Autodesk Inventor part; units mm, degrees
ref_plane "YZ Plane" through (0, 0, 0) normal (1, 0, 0) x (0, 1, 0)
ref_plane "XZ Plane" through (0, 0, 0) normal (0, 1, 0) x (-1, 0, 0)
ref_plane "XY Plane" through (0, 0, 0) normal (0, 0, 1) x (1, 0, 0)
sketch "Sketch1" plane through (0, 0, 0) normal (1, 0, 0) x (0, 1, 0)
  line L0 (-19.05, 19.05) -> (19.05, 19.05)
  line L1 (19.05, 19.05) -> (19.05, -19.05)
  line L2 (19.05, -19.05) -> (-19.05, -19.05)
  line L3 (-19.05, -19.05) -> (-19.05, 19.05)
  line L4 (-19.05, 19.05) -> (19.05, -19.05) construction
  line L5 (19.05, 19.05) -> (-19.05, -19.05) construction
  line L6 (19.05, 19.05) -> (-19.05, -19.05)
  line L7 (19.05, -19.05) -> (-19.05, 19.05)
  line L8 (0, 0) -> (0, -19.05)
  line L9 (0, 0) -> (0, 19.05)
  circle A0 centre (0, 9.525) radius 3.81
  circle A1 centre (0, -9.525) radius 3.81
  dimension "d0" = 38.1
  dimension "d1" = 38.1
  dimension "d2" = 7.62
  dimension "d3" = 7.62
  dimension "d4" = 19.05
extrude "Extrusion1" add sketch "Sketch1" along normal blind 38.1 contours L7 L6 L3 | L0 L9 A0 L7 | L0 L6 L9 A0 | L6 L8 A1 L2 | L6 L1 L7 | L7 L2 L8 A1
sketch "Sketch2" plane through (0, -19.05, -19.05) normal (0, -1, 0) x (1, 0, 0)
  line L0 (38.1, 0) -> (38.1, 38.1)
  line L1 (0, 0) -> (38.1, 0)
  line L2 (38.1, 38.1) -> (38.1, 0)
  line L3 (38.1, 0) -> (0, 0)
  line L4 (0, 0) -> (0, 38.1)
  line L5 (0, 0) -> (0, 38.1)
  line L6 (0, 38.1) -> (38.1, 38.1)
  line L7 (0, 38.1) -> (38.1, 38.1)
  line L8 (0, 0) -> (38.1, 38.1)
  line L9 (38.1, 0) -> (0, 38.1)
  circle A0 centre (19.05, 19.05) radius 12.5
  point P0 (0, 19.05)
  dimension "d7" = 25
extrude "Extrusion2" cut sketch "Sketch2" against normal blind 15 contours A0 L8 L9 | L9 L8 A0 | L8 L9 A0 | A0 L9 L8
fillet "Fillet1" radius 2 1 edges at (19.05, 19.05, 19.05)
fillet "Fillet2" radius 2 1 edges at (19.05, 19.05, -19.05)
properties part number "cube fixation2"
Check sheet for the modelled part. Datum: model origin and axes. Units: mm. A direction names the side the tool comes from. Round coordinates to 2 decimals unless told otherwise and drop trailing zeros. Order: outer loops, then holes, each group sorted by start corner. A loop starts at its lowest first (then second) coordinate and runs counter-clockwise, first axis right, second up.
1) Section check D-D (x = 33). Record the boundary of the cut face in (y, z) (3 decimals).
2) Section check C-C (z = 0). Record the boundary of the cut face in (x, y).
3) Section check B-B (y = -11). Record the boundary of the cut face in (x, z).
4) Section check A-A (y = 0). Record the boundary of the cut face in (x, z) (3 decimals).
5) Mould release check, pull along Z, two halves, no side actions. Record for faces 1 (the flat face through (19, -1, -19.05)), 2 (the cylindrical face through (19.32, 18.48, 18.45)), 3 (the cylindrical face through (18.8, -0.8, -5.8)): +Z half, -Z half, draft (parallel to the pull), parting line (faces both ways), or undercut.
6) Go/stop test with flat-tipped pins: pin 1 Ø1 at (x, z) = (26.5, -8.5) entering from -Y; pin 2 Ø1.5 at (y, z) = (2.5, 9) entering from -X. Record where each tip stops, or that it passes through.
7) Tool access check on faces 4 (the flat face through (19, -1, 19.05)), 5 (the cylindrical face through (6.562, -11.655, 0.55)). Record the directions out of +Z, -Z, +X, -X, +Y, -Y that give a thin tool (end or side, any length) a straight path to the whole face; none if there is none.
8) Scan lines: line 1 (Z direction, x = 30, y = 0) (3 decimals); line 2 (Z direction, x = 19, y = -12); line 3 (Y direction, x = 5, z = -9.5). Record each from-to range of solid material in increasing order.
Result:
1. outline: (-19.05, -19.05) - (17.05, -19.05) arc R2 ccw to (19.05, -17.05) - (19.05, 17.05) arc R2 ccw to (17.05, 19.05) - (-19.05, 19.05) - close; hole circle Ø7.62 at (0, -9.525); hole circle Ø7.62 at (0, 9.525)
2. outline: (0, -19.05) - (6.55, -19.05) - (6.55, -4.05) - (31.55, -4.05) - (31.55, -19.05) - (38.1, -19.05) - (38.1, 19.05) - (0, 19.05) - close
3. outline: (0, -19.05) - (38.1, -19.05) - (38.1, 19.05) - (0, 19.05) - close; hole circle Ø25 at (19.05, 0)
4. outline: (0, -19.05) - (38.1, -19.05) - (38.1, -13.335) - (0, -13.335) - close; (0, -5.715) - (38.1, -5.715) - (38.1, 5.715) - (0, 5.715) - close; (0, 13.335) - (38.1, 13.335) - (38.1, 19.05) - (0, 19.05) - close
5. face 1: -Z half
5. face 2: +Z half
5. face 3: undercut
6. pin 1: stops at y = -4.05
6. pin 2: passes through
7. face 4: +Z, +X, -X, +Y, -Y
7. face 5: -Y
8. line 1: z = -19.05 to -13.335, -5.715 to 5.715, 13.335 to 19.05
8. line 2: z = -19.05 to -12.5, 12.5 to 19.05
8. line 3: y = -19.05 to -3.81, 3.81 to 19.05
